Autodesk Inventor part; units mm, degrees
ref_plane "YZ Plane" through (0, 0, 0) normal (1, 0, 0) x (0, 1, 0)
ref_plane "XZ Plane" through (0, 0, 0) normal (0, 1, 0) x (-1, 0, 0)
ref_plane "XY Plane" through (0, 0, 0) normal (0, 0, 1) x (1, 0, 0)
sketch "Sketch1" plane through (0, 0, 0) normal (0, 0, 1) x (1, 0, 0)
  circle A0 centre (-57.8697, -2.8503) radius 2.0955
  circle A1 centre (-7.0697, -2.8503) radius 2.0955
  circle A2 centre (31.0303, -2.8503) radius 2.0955
  circle A3 centre (69.1303, -2.8503) radius 2.0955
  arc A4 (-62.7892, 5.306) -> (-57.8697, -12.3753) centre (-57.8697, -2.8503) ccw
  arc A5 (-30.9405, 22.3406) -> (-35.7494, 21.615) centre (-32.4697, 16.1775) ccw
  arc A6 (69.1303, -12.3753) -> (69.1303, 6.6747) centre (69.1303, -2.8503) ccw
  line L0 (-57.8697, -12.3753) -> (69.1303, -12.3753)
  line L1 (-62.7892, 5.306) -> (-35.1787, 21.9592)
  line L2 (69.1303, 6.6747) -> (38.4028, 6.6747)
  line L3 (-30.9405, 22.3406) -> (26.1686, 8.1699)
  arc A7 (26.1686, 8.1699) -> (38.4028, 6.6747) centre (38.4028, 57.4747) ccw
  circle A8 centre (-32.4697, 16.1775) radius 2.0955
  point P0 (0, 0)
  dimension "d0" = 4.191
  dimension "d1" = 4.191
  dimension "d2" = 4.191
  dimension "d3" = 4.191
  dimension "d4" = 50.8
  dimension "d5" = 4.191
extrude "Extrusion1" add sketch "Sketch1" along normal blind 1.5875
sketch "Sketch2" plane through (-7.0697, -2.8503, 0) normal (0, 0, -1) x (-1, 0, 0)
  circle A0 centre (25.4, 0) radius 2.0955
  point P0 (-7.0697, 2.8503)
  dimension "d8" = 4.191
extrude "Extrusion2" cut sketch "Sketch2" against normal blind 1.5875
sketch "Sketch3" plane through (-7.0697, -2.8503, 0) normal (0, 0, -1) x (-1, 0, 0)
  line L0 (-21.6825, 26.7893) -> (-14.3342, 17.6126)
  line L1 (-30.135, 24.3239) -> (-31.2875, 13.6514)
  line L2 (-33.2384, 11.0202) -> (23.8707, 25.1909)
  line L3 (-33.6796, 10.9107) -> (-33.2384, 11.0202)
  arc A0 (-33.6796, 10.9107) -> (-31.2875, 13.6514) centre (-34.4442, 13.9923) ccw
  line L4 (23.8707, 25.1909) -> (-11.0912, 16.5156)
  arc A1 (-14.3342, 17.6126) -> (-11.0912, 16.5156) centre (-11.8558, 19.5972) ccw
  circle A2 centre (-25.4, 23.8125) radius 2.0828
  arc A3 (-21.6825, 26.7893) -> (-30.135, 24.3239) centre (-25.4, 23.8125) ccw
  point P0 (-7.0697, 2.8503)
  point P1 (-13.3897, 15.9453)
  point P2 (-13.0638, 16.0262)
  dimension "d19" = 3.175
  dimension "d20" = 3.175
  dimension "d21" = 4.1656
extrude "Extrusion3" add sketch "Sketch3" against normal blind 1.5875
sketch "Sketch5" plane through (69.1303, -2.8503, 1.5875) normal (0, 0, 1) x (1, 0, 0)
  circle A0 centre (25.4, 0) radius 2.0955
  arc A1 (25.4, -9.525) -> (25.4, 9.525) centre (25.4, 0) ccw
  line L0 (25.4, 9.525) -> (0, 9.525)
  arc A2 (0, -9.525) -> (0, 9.525) centre (0, 0) ccw
  line L1 (0, -9.525) -> (25.4, -9.525)
  point P0 (-69.1303, 2.8503)
  dimension "d26" = 4.191
extrude "Extrusion5" add sketch "Sketch5" against normal blind 1.5875
properties part number "intake_gusset" material "Acetal Resin, White"
Read the model definition and answer for the solid it produces. Units are mm, in the model's axes. A direction names the side the tool comes from. Round coordinates to 2 decimals unless told otherwise and drop trailing zeros. Order: outer loops, then holes, each group sorted by start corner. A loop starts at its lowest first (then second) coordinate and runs counter-clockwise, first axis right, second up.
1) The part is cut by section A-A on x = 31. Write down the section's boundary in (y, z), plus the area to 3 significant figures.
2) The part is cut by section D-D on y = -10. Write down the section's boundary in (x, z), plus the area to 3 significant figures.
3) Straight lines are drawn through the part: L1, parallel to Y at x = 94.5, z = 0.5; L2, parallel to Y at x = 55, z = 0.15; L3, parallel to Y at x = -59.5, z = 0.15. For each, find the intervals that lie inside material, in ascending order.
4) The part is cut by section B-B on z = 0.5. Give the number of separate pieces and of enclosed holes in the cut face, plus the area to 3 significant figures.
5) The mould has two halves that part along Y. Classify faces 1 (the face through (19.588, 25.556, 0.783)), 2 (the face through (-67, -5.57, 0.78)), 3 (the face through (-5.07, -3.48, 0.78)): released by +Y, released by -Y, zero draft, split by the parting line, or undercut.
6) For faces 4 (the face through (10.99, 19.415, 0.783)), 5 (the face through (-49.459, 13.346, 0.783)), determine the directions among +Z, -Z, +X, -X, +Y, -Y from which every point of the face is accessible in a straight line to the end or side of a thin tool.
7) The part is cut by section C-C on x = 49. Write down the section's boundary in (y, z), plus the area to 3 significant figures.
8) A flat-ended cylindrical pin translates along its axis: pin 1 (3.5 mm diameter, centred on x = -7.07, y = -2.85, fed in from +Z). Find the tip coordinate at first contact, or state that the pin passes through.
Resolved:
1. outline: (-12.38, 0) - (-4.95, 0) - (-4.95, 1.59) - (-12.38, 1.59) - close; (-0.76, 0) - (7.22, 0) - (7.22, 1.59) - (-0.76, 1.59) - close
1. area: 24.5 mm2
2. outline: (-64.16, 0) - (100.82, 0) - (100.82, 1.59) - (-64.16, 1.59) - close
2. area: 262 mm2
3. L1: y = -12.38 to -4.95, -0.76 to 6.67
3. L2: y = -12.38 to 6.67
3. L3: y = -12.23 to -4.17, -1.53 to 7.29
4. separate pieces: 1
4. enclosed holes: 8
4. area: 4,030 mm2
5. face 1: released by +Y
5. face 2: split by the parting line
5. face 3: undercut
6. face 4: +Z, -Z, +Y
6. face 5: +Z, -Z, -X, +Y
7. outline: (-12.38, 0) - (6.67, 0) - (6.67, 1.59) - (-12.38, 1.59) - close
7. area: 30.2 mm2
8. pin 1: passes through
